Could you check a few things on this drawing? It's one solid part, dimensions in mm from its lowest x, y, z. A direction names the side the tool comes from. Give positions to 0.01 mm unless a question says otherwise; leave off trailing zeros. Loops run counter-clockwise (first coordinate to the right, second up) from the corner with the lowest first, then second, coordinate; pieces in that order, holes last. Notation, with made-up numbers: (-16.75, 77.25) - (25.25, 77.25) arc R21 cw to (25.25, 114.25) - close; hole circle Ø1 at (-22.75, -1). An arc over 180 degrees is marked (long way). Put each result on its own line as item: value. Start each with the question number.
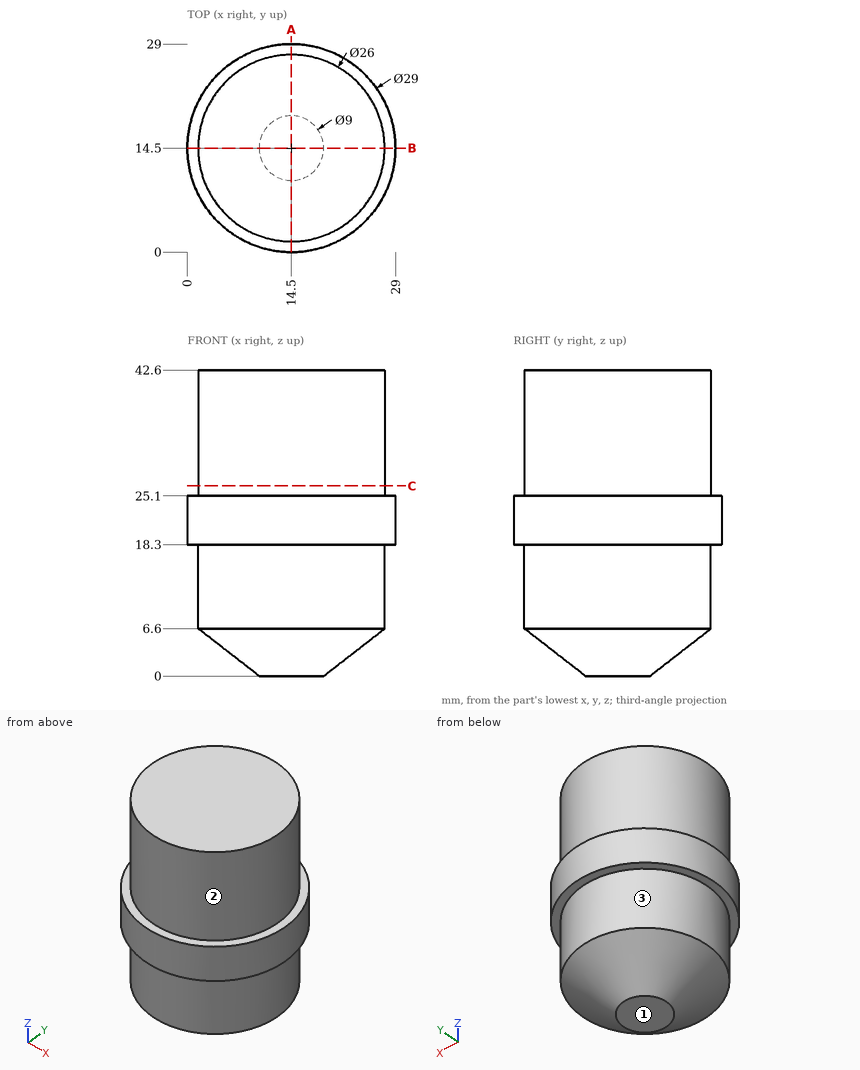
1) Suppose I cut it at A-A on x = 14.5. Please give me the cut outline in (y, z).
2) Which directions (+Z, -Z, +X, -X, +Y, -Y) give clear straight access to the entire face, cutting with the end or side of a thin tool? Please do the marked faces 1, 2 and 3.
3) I'm going to push flat-ended pins straight in: P1, Ø1.5, axis at x = 20.5, z = 29.5, coming from the -Y side; P2, Ø1.5, axis at y = 13.5, z = 19, coming from the +X side; P3, Ø1, axis at x = 17, z = 28.5, coming from the -Y side. Where does each tip first touch, or does it pass through?
4) Suppose I cut it at C-C on z = 26.5. Please give me the cut outline in (x, y), plus the area to 3 significant figures.
5) I need wall thicknesses on line 1 (X direction, y = 14.25, z = 9); line 2 (X direction, y = 4, z = 30); line 3 (Z direction, x = 8.5, y = 20.5). Which ranges of each line are inside material? Lowest first, please.
Ans:
1. outline: (0, 18.3) - (1.5, 18.3) - (1.5, 6.6) - (10, 0) - (19, 0) - (27.5, 6.6) - (27.5, 18.3) - (29, 18.3) - (29, 25.1) - (27.5, 25.1) - (27.5, 42.6) - (1.5, 42.6) - (1.5, 25.1) - (0, 25.1) - close
2. face 1: -Z, +X, -X, +Y, -Y
2. face 2: +Z
2. face 3: -Z
3. P1: stops at y = 2.61
3. P2: stops at x = 29
3. P3: stops at y = 1.65
4. outline: circle Ø26 at (14.5, 14.5)
4. area: 531 mm²
5. line 1: x = 1.5 to 27.5
5. line 2: x = 6.84 to 22.16
5. line 3: z = 3.09 to 42.6
